```python
from build123d import *

# Parameters (mm, degrees)
EXTRUDE_1_DEPTH  = 15
CHAMFER_1_SIZE   = 2
CHAMFER_2_SIZE   = 0.5
MIRROR_START     = -8.660254038
MIRROR_2_DEPTH   = 2.193931023
MIRROR_START_2   = 6.466323015
MIRROR_2_2_DEPTH = 2.193931023


# Read off the part's stored shape, not the designer's step: 镜向2
with BuildPart() as part:
    # 草图1 → 凸台-拉伸1 (new, symmetric)
    with BuildSketch(Plane.XY):
        Polygon((-3, 0), (3, 0), (3, -2), (5.3, -2), (5.3, -6), (-5.3, -6), (-5.3, -2), (-3, -2), align=None)
    extrude(amount=EXTRUDE_1_DEPTH, both=True)

    # 倒角1
    chamfer_1_edges = [part.edges().sort_by_distance(p)[0] for p in [
        (5.3, -6, 0),
        (-5.3, -6, 0),
    ]]
    chamfer(chamfer_1_edges, length=CHAMFER_1_SIZE)

    # 倒角2
    chamfer_2_edges = [part.edges().sort_by_distance(p)[0] for p in [
        (-3, -1, 15),
        (-4.15, -2, 15),
        (-5.3, -3, 15),
        (5.3, -3, 15),
        (4.15, -2, 15),
        (3, -1, 15),
    ]]
    chamfer(chamfer_2_edges, length=CHAMFER_2_SIZE)

    # 镜向2 outline → 镜向2 (cut)
    with BuildSketch(Plane(origin=(0, 0, 0), x_dir=(0.8164965809277261, -0.4082482904638631, -0.4082482904638625), z_dir=(0.5773502691896255, 0.5773502691896263, 0.5773502691896255)).offset(MIRROR_START)):
        Polygon((9.185586535, 8.838834765), (11.063528672, 8.838834765), (11.880025252, 7.424621202), (12.702530685, 6), (13, 6), (13, 12), (7.360486936, 12), (8.164965809, 10.606601718), align=None)
    extrude(amount=MIRROR_2_DEPTH, mode=Mode.SUBTRACT)

    # Mirror 2 2 outline → Mirror 2 2 (cut)
    with BuildSketch(Plane(origin=(0, 0, 0), x_dir=(0.816496580927727, 0.4082482904638606, 0.4082482904638635), z_dir=(0.5773502691896244, -0.5773502691896244, -0.5773502691896285)).offset(MIRROR_START_2)):
        Polygon((-8.164965809, -10.606601718), (-9.185586535, -8.838834765), (-11.063528672, -8.838834765), (-11.880025252, -7.424621202), (-12.702530685, -6), (-13, -6), (-13, -12), (-7.360486936, -12), align=None)
    extrude(amount=MIRROR_2_2_DEPTH, mode=Mode.SUBTRACT)


solid = part.part
```
CAD build for the part. Positions are in the model's coordinates, mm. A direction names the side the tool comes from. Round coordinates to 2 decimals unless told otherwise and drop trailing zeros. Order: outer loops, then holes, each group sorted by start corner. A loop starts at its lowest first (then second) coordinate and runs counter-clockwise, first axis right, second up. Notation, with made-up numbers: (17, 72.25) - (22, 72.25) arc R31 ccw to (22, 102.25) - close; hole circle Ø11 at (17.5, 65.5). An arc over 180 degrees is marked (long way). Answer in a Markdown table with one row per item. Add a question column.
(1) Band-saw the part on D-D on x = 4. List the corners of the cut face in (y, z).
(2) 3-axis set-ups, long thin cutter, end or side, ignore diameter. For faces 4 (the face through (-4.3, -5, 0.2)), 5 (the face through (4, -2, 0)), 6 (the face through (-4, -2, 0)): which of +Z, -Z, +X, -X, +Y, -Y reach the whole face in a straight line?
(3) Band-saw the part on C-C on z = -8. List the corners of the cut face in (x, y), and give its area (3 significant figures).
(4) Drop flat-ended pins along their axis: pin 1 Ø0.7 at (x, z) = (-4, -5) entering from +Y; pin 2 Ø1 at (x, z) = (4, 11.5) entering from -Y; pin 3 Ø2 at (y, z) = (-0.5, -2) entering from -X. Give the stop position or say it passes through.
(5) Band-saw the part on A-A on y = -0.85. List the corners of the cut face in (x, z), and give its area (4 significant figures).
(6) Mould opens along X. For faces 1 (the face through (4.3, -5, 0.2)), 2 (the face through (0, -6, 0)), 3 (the face through (-3, -1, 0)) say: +X half, -X half, draft (parallel to the pull), parting line (faces both ways), or undercut.
(7) Band-saw the part on B-B on x = -4.5. List the corners of the cut face in (y, z).
(8) Probe L1, parallel to Y at x = 4, z = -8.5; L2, parallel to X at y = -0.9, z = -4; L3, parallel to X at y = -4.25, z = 6. List the from-to ranges inside material, lowest first. Write a range as [from, to].
Data:
| question | item | result |
|---|---|---|
| 1 | outline | (-5.3, -15) - (-2.5, -15) - (-2, -14.5) - (-2, 14.5) - (-2.5, 15) - (-5.3, 15) - close |
| 2 | face 4 | +Z, -Z, -X, -Y |
| 2 | face 5 | +Z, -Z, +X, +Y |
| 2 | face 6 | +Z, -Z, -X, +Y |
| 3 | outline | (-5.3, -4) - (-3.3, -6) - (3.3, -6) - (5.3, -4) - (5.3, -2) - (3, -2) - (3, 0) - (-3, 0) - (-3, -2) - (-5.3, -2) - close |
| 3 | area | 50.4 mm^2 |
| 4 | pin 1 | stops at y = -2 |
| 4 | pin 2 | stops at y = -5.8 |
| 4 | pin 3 | stops at x = -3 |
| 5 | outline | (-3, -14.5) - (-2.5, -15) - (2.5, -15) - (3, -14.5) - (3, 14.5) - (2.5, 15) - (-2.5, 15) - (-3, 14.5) - close |
| 5 | area | 179.5 mm^2 |
| 6 | face 1 | +X half |
| 6 | face 2 | draft |
| 6 | face 3 | -X half |
| 7 | outline | (-4.8, -15) - (-2.5, -15) - (-2, -14.5) - (-2, 14.5) - (-2.5, 15) - (-4.8, 15) - close |
| 8 | L1 | y = [-5.3, -2] |
| 8 | L2 | x = [-3, 3] |
| 8 | L3 | x = [-5.05, 5.05] |
